Check sheet for the drawn part. Datum: minimum x, y, z corner. Units: mm. Round coordinates to 2 decimals unless told otherwise and drop trailing zeros. Order: outer loops, then holes, each group sorted by start corner. A loop starts at its lowest first (then second) coordinate and runs counter-clockwise, first axis right, second up. Notation, with made-up numbers: (15, 27) -> (72, 27) arc R25 cw to (72, 51) -> close; hole circle Ø8 at (57.5, 7.25). An arc over 180 degrees is marked (long way). Answer in a Markdown table with one row per item.
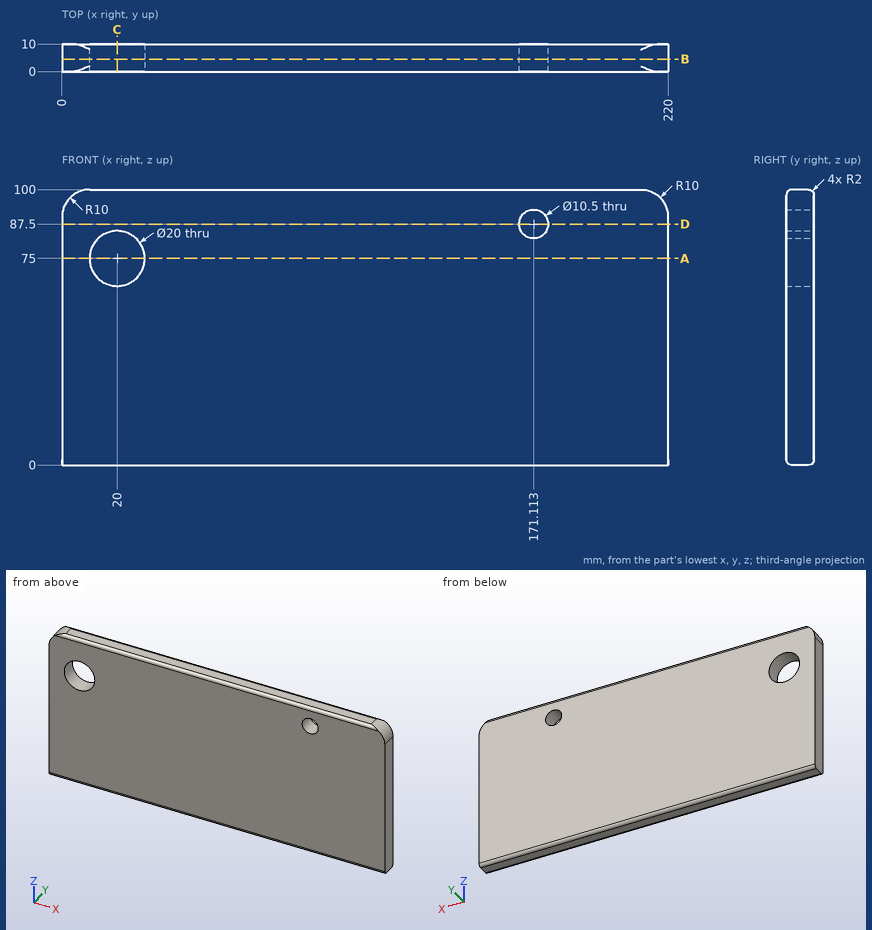
(1) Section check D-D on z = 87.5. Record the boundary of the cut face in (x, y), plus the area to 4 significant figures.
Solutions:
| item | result |
|---|---|
| outline | (0, 0) -> (165.86, 0) -> (165.86, 10) -> (0, 10) -> close; (176.36, 0) -> (220, 0) -> (220, 10) -> (176.36, 10) -> close |
| area | 2,095 mm^2 |
(2) Section check A-A on z = 75. Record the boundary of the cut face in (x, y).
Solutions:
| item | result |
|---|---|
| outline | (0, 0) -> (10, 0) -> (10, 10) -> (0, 10) -> close; (30, 0) -> (220, 0) -> (220, 10) -> (30, 10) -> close |
(3) Section check C-C on x = 20. Record the boundary of the cut face in (y, z).
Solutions:
| item | result |
|---|---|
| outline | (0, 2) arc R2 ccw to (2, 0) -> (8, 0) arc R2 ccw to (10, 2) -> (10, 65) -> (0, 65) -> close; (0, 85) -> (10, 85) -> (10, 98) arc R2 ccw to (8, 100) -> (2, 100) arc R2 ccw to (0, 98) -> close |
(4) Section check B-B on y = 4.5. Record the boundary of the cut face in (x, z), plus the area to 3 significant figures.
Solutions:
| item | result |
|---|---|
| outline | (0, 0) -> (220, 0) -> (220, 90) arc R10 ccw to (210, 100) -> (10, 100) arc R10 ccw to (0, 90) -> close; hole circle Ø20 at (20, 75); hole circle Ø10.5 at (171.11, 87.5) |
| area | 21,600 mm^2 |
(5) Scan lines: probe 1 along Z at (x, y) = (20, 2.5); probe 2 along X at (y, z) = (1.75, 66.5); probe 3 along X at (y, z) = (9.25, 81.5). Record each from-to range of solid material in increasing order. Write a range as from..to.
Solutions:
| item | result |
|---|---|
| probe 1 | 0..65, 85..100 |
| probe 2 | 0..14.73, 25.27..220 |
| probe 3 | 0..12.4, 27.6..220 |
